Part model, mm, in its own coordinate system. Face numbers are marked on the shaded views. A direction names the side the tool comes from. Give positions to 0.01 mm unless a question says otherwise; leave off trailing zeros. Order: outer loops, then holes, each group sorted by start corner. A loop starts at its lowest first (then second) coordinate and runs counter-clockwise, first axis right, second up. Notation, with made-up numbers: (11.5, -22.75) - (30.5, -22.75) arc R22 cw to (30.5, -12.75) - close; hole circle Ø3 at (79.25, -25). An arc over 180 degrees is marked (long way). Use a Markdown table: item, result. Add a question column.
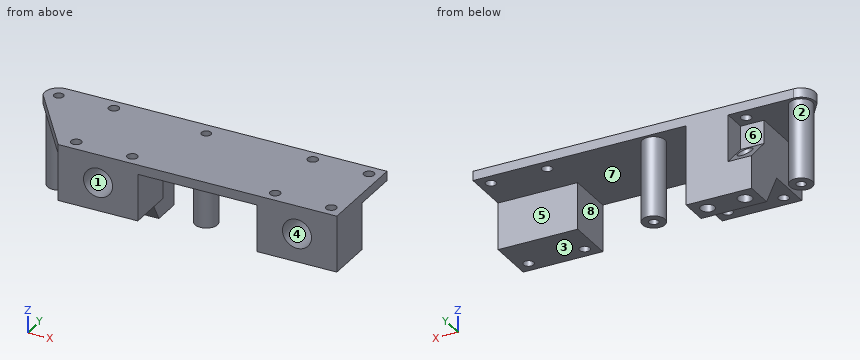
from build123d import *

# Parameters (mm, degrees)
SKETCH056_R     = 1.1
SKETCH056_R_2   = 1
PAD026_DEPTH    = 2
SKETCH072_W     = 17
SKETCH072_H     = 10
SKETCH072_R     = 1.1
PAD031_DEPTH    = 10
SKETCH073_R     = 2.4
SKETCH073_R_2   = 1
SKETCH073_W     = 14
SKETCH073_H     = 10
SKETCH073_R_3   = 1.5
PAD032_DEPTH    = 17
POCKET035_DEPTH = 14
POCKET036_DEPTH = 5
SKETCH076_R     = 3.1
POCKET037_DEPTH = 8


with BuildPart() as part:
    # Sketch056 → Pad026 (new body)
    with BuildSketch(Plane(origin=(-8.5, 115, 6), x_dir=(1, 0, 0), z_dir=(0, 0, -1))):
        with BuildLine():
            Line((0, 0), (59.5, 0))
            Line((59.5, 0), (59.5, 20))
            Line((59.5, 20), (0, 20))
            Line((0, 20), (-11.819078, 4.02606))
            ThreePointArc((-11.819078, 4.02606), (-11.457456, 1.279271), (-9, 0))
            Line((0, 0), (-9, 0))
        make_face()
        with Locations((2.5, 17.5)):
            Circle(SKETCH056_R, mode=Mode.SUBTRACT)
        with Locations((14.5, 17.5)):
            Circle(SKETCH056_R, mode=Mode.SUBTRACT)
        with Locations((45, 17.5)):
            Circle(SKETCH056_R, mode=Mode.SUBTRACT)
        with Locations((45, 2.5)):
            Circle(SKETCH056_R, mode=Mode.SUBTRACT)
        with Locations((57, 17.5)):
            Circle(SKETCH056_R, mode=Mode.SUBTRACT)
        with Locations((57, 2.5)):
            Circle(SKETCH056_R, mode=Mode.SUBTRACT)
        with Locations((2.5, 2.5)):
            Circle(SKETCH056_R, mode=Mode.SUBTRACT)
        with Locations((22.5, 3)):
            Circle(SKETCH056_R_2, mode=Mode.SUBTRACT)
        with Locations((-9, 3)):
            Circle(SKETCH056_R_2, mode=Mode.SUBTRACT)
    extrude(amount=PAD026_DEPTH)

    # Sketch072 → Pad031 (new body)
    with BuildSketch(Plane(origin=(-8.5, 115, 4), x_dir=(1, 0, 0), z_dir=(0, 0, -1))):
        with Locations((8.5, 15)):
            Rectangle(SKETCH072_W, SKETCH072_H)
        with Locations((2.5, 17.5)):
            Circle(SKETCH072_R, mode=Mode.SUBTRACT)
        with Locations((14.5, 17.5)):
            Circle(SKETCH072_R, mode=Mode.SUBTRACT)
        with Locations((51, 15)):
            Rectangle(SKETCH072_W, SKETCH072_H)
        with Locations((45, 17.5)):
            Circle(SKETCH072_R, mode=Mode.SUBTRACT)
        with Locations((57, 17.5)):
            Circle(SKETCH072_R, mode=Mode.SUBTRACT)
    extrude(amount=PAD031_DEPTH)

    # Sketch073 → Pad032 (new body)
    with BuildSketch(Plane(origin=(-8.5, 115, 4), x_dir=(1, 0, 0), z_dir=(0, 0, -1))):
        with Locations((22.5, 3)):
            Circle(SKETCH073_R)
        with Locations((22.5, 3)):
            Circle(SKETCH073_R_2, mode=Mode.SUBTRACT)
        with Locations((-9, 3)):
            Circle(SKETCH073_R)
        with Locations((-9, 3)):
            Circle(SKETCH073_R_2, mode=Mode.SUBTRACT)
        with Locations((7, 5)):
            Rectangle(SKETCH073_W, SKETCH073_H)
        with Locations((11, 3)):
            Circle(SKETCH073_R_3, mode=Mode.SUBTRACT)
        with Locations((3, 3)):
            Circle(SKETCH073_R_3, mode=Mode.SUBTRACT)
    extrude(amount=PAD032_DEPTH)

    # Sketch074 → Pocket035 (cut)
    with BuildSketch(Plane(origin=(-8.5, 115, 6), x_dir=(0, 1, 0), z_dir=(-1, 0, 0))):
        Polygon((-10, 12), (-10, 19), (-6, 19), align=None)
    extrude(amount=-POCKET035_DEPTH, mode=Mode.SUBTRACT)

    # Sketch075 → Pocket036 (cut)
    with BuildSketch(Plane(origin=(-8.5, 115, 6), x_dir=(0, 1, 0), z_dir=(-1, 0, 0))):
        Polygon((0, 2), (0, 12), (-5, 7), (-5, 2), align=None)
    extrude(amount=-POCKET036_DEPTH, mode=Mode.SUBTRACT)

    # Sketch076 → Pocket037 (cut)
    with BuildSketch(Plane(origin=(-8.5, 95, 6), x_dir=(-1, 0, 0), z_dir=(0, -1, 0))):
        with Locations((-8.5, 6)):
            Circle(SKETCH076_R)
        with Locations((-51, 6)):
            Circle(SKETCH076_R)
    extrude(amount=-POCKET037_DEPTH, mode=Mode.SUBTRACT)


solid = part.part
1. Cut at D-D (x = 48.5). Write the cut outline in (y, z), plus the area to 3 significant figures.
2. Pin check, flat tips, straight feed: P1, Ø1, axis at x = 39, z = 2.5, coming from the +Y side; P2, Ø2.5, axis at x = -6, z = 2.5, coming from the +Y side; P3, Ø1, axis at x = -0.5, z = -9.5, coming from the -Y side. Stop position of each tip, or through.
3. Mould opens along Z. For the marked faces 1, 2 and 3 say: released by +Z, released by -Z, zero draft, split by the parting line, or undercut.
4. Cut at B-B (y = 97.5). Write the cut outline in (x, z), plus the area to 3 significant figures.
5. Tool access for the marked faces 4, 5, 6, 7 and 8: list every direction of +Z, -Z, +X, -X, +Y, -Y with a clear straight run to the whole face (end or side of a thin tool).
6. Cut at A-A (z = 0). State how many separate pieces and enclosed holes the cut face has, plus the area to 3 significant figures.
7. Drill centre lines: probe 1 along Y at (x, z) = (-6, 5); probe 2 along X at (y, z) = (100.5, 0); probe 3 along X at (y, z) = (112.5, 5.1). Where is each one in solid material? Low to high. Write a range as [from, to].
Responses:
| question | item | result |
|---|---|---|
| 1 | outline | (95, -6) - (96.4, -6) - (96.4, 6) - (95, 6) - close; (98.6, -6) - (105, -6) - (105, 4) - (111.4, 4) - (111.4, 6) - (98.6, 6) - close; (113.6, 4) - (115, 4) - (115, 6) - (113.6, 6) - close |
| 1 | area | 109 mm² |
| 2 | P1 | stops at y = 105 |
| 2 | P2 | stops at y = 110 |
| 2 | P3 | stops at y = 106.71 |
| 3 | face 1 | undercut |
| 3 | face 2 | zero draft |
| 3 | face 3 | released by -Z |
| 4 | outline | (-10.35, 4) - (-8.5, 4) - (-8.5, -6) - (-7.1, -6) - (-7.1, 6) - (-10.35, 6) - close; (-4.9, -6) - (4.9, -6) - (4.9, 6) - (-4.9, 6) - close; (7.1, -6) - (8.5, -6) - (8.5, 4) - (34, 4) - (34, -6) - (35.4, -6) - (35.4, 6) - (7.1, 6) - close; (37.6, -6) - (47.4, -6) - (47.4, 6) - (37.6, 6) - close; (49.6, -6) - (51, -6) - (51, 6) - (49.6, 6) - close; hole circle Ø6.2 at (0, 0); hole circle Ø6.2 at (42.5, 0) |
| 4 | area | 297 mm² |
| 5 | face 4 | -Y |
| 5 | face 5 | -Z, +X, +Y |
| 5 | face 6 | +Y |
| 5 | face 7 | -Z |
| 5 | face 8 | -Z, +Y, -Y |
| 6 | separate pieces | 4 |
| 6 | enclosed holes | 7 |
| 6 | area | 363 mm² |
| 7 | probe 1 | y = [95, 96.4], [98.6, 111.4], [113.6, 115] |
| 7 | probe 2 | x = [-8.5, -3.1], [3.1, 8.5], [34, 39.4], [45.6, 51] |
| 7 | probe 3 | x = [-20.46, -18.37], [-16.63, -7.1], [-4.9, 13.13], [14.87, 35.4], [37.6, 47.4], [49.6, 51] |
